```python
from build123d import *

# Parameters (mm, degrees)
F0_W     = 12.4
F0_H     = 29.8
F1_DEPTH = 12
F2_W     = 58.4
F2_H     = 12
F2_R     = 2.5
F3_DEPTH = 5
F4_R     = 5
F5_R     = 5
F6_R     = 5
F7_R     = 4.75
F8_DEPTH = 2
F9_R     = 1
F10_R    = 5


# Not quite as in the source:
# - a feature names something its author has since deleted; it is built from what else it names


with BuildPart() as f1:
    # F0 (on Top) → F1 (new body)
    with BuildSketch(Plane.XY):
        with BuildLine():
            ThreePointArc((-8.2, 0), (0, 8.2), (8.2, 0))
            Line((8.2, 0), (11.2, 0))
            Line((11.2, 0), (11.2, 52))
            Line((11.2, 52), (0, 52))
            Line((0, 52), (-11.2, 52))
            Line((-11.2, 52), (-11.2, 0))
            Line((-11.2, 0), (-8.2, 0))
        make_face()
        with Locations((0, 30.1)):
            Rectangle(F0_W, F0_H, mode=Mode.SUBTRACT)
        with BuildLine():
            Line((11.2, 0), (8.2, 0))
            ThreePointArc((8.2, 0), (0, -8.2), (-8.2, 0))
            Line((-8.2, 0), (-11.2, 0))
            Line((-11.2, 0), (-11.2, -12.2))
            Line((-11.2, -12.2), (0, -12.2))
            Line((0, -12.2), (11.2, -12.2))
            Line((11.2, -12.2), (11.2, 0))
        make_face()
        with BuildLine():
            Line((11.2, 0), (8.2, 0))
            ThreePointArc((8.2, 0), (0, -8.2), (-8.2, 0))
            Line((-8.2, 0), (-11.2, 0))
            Line((-11.2, 0), (-11.2, -12.2))
            Line((-11.2, -12.2), (0, -12.2))
            Line((0, -12.2), (11.2, -12.2))
            Line((11.2, -12.2), (11.2, 0))
        make_face()
    extrude(amount=F1_DEPTH)

    # F2 (on face) → F3 (join)
    with BuildSketch(Plane(origin=(0, 52, 0), x_dir=(-1, 0, 0), z_dir=(0, 1, 0))):
        with Locations((0, 6)):
            Rectangle(F2_W, F2_H)
        with Locations((-21.7, 6)):
            Circle(F2_R, mode=Mode.SUBTRACT)
        with Locations((21.7, 6)):
            Circle(F2_R, mode=Mode.SUBTRACT)
    extrude(amount=F3_DEPTH)

    # F4
    f4_edges = [f1.edges().sort_by_distance(p)[0] for p in [
        (-11.2, -12.2, 6),
        (11.2, -12.2, 6),
    ]]
    fillet(f4_edges, radius=F4_R)

    # F5
    f5_edges = [f1.edges().sort_by_distance(p)[0] for p in [
        (11.2, 52, 6),
        (-11.2, 52, 6),
    ]]
    fillet(f5_edges, radius=F5_R)

    # F6
    f6_edges = [f1.edges().sort_by_distance(p)[0] for p in [
        (-29.2, 54.5, 12),
        (-29.2, 54.5, 0),
        (29.2, 54.5, 0),
        (29.2, 54.5, 12),
    ]]
    fillet(f6_edges, radius=F6_R)

    # F7 (on face) → F8 (cut)
    with BuildSketch(Plane.XZ.offset(-52)):
        with Locations((21.7, 6)):
            Circle(F7_R)
        with Locations((-21.7, 6)):
            Circle(F7_R)
    extrude(amount=-F8_DEPTH, mode=Mode.SUBTRACT)

    # F9
    f9_edges = [f1.edges().sort_by_distance(p)[0] for p in [
        (8.2, 0, 12),
    ]]
    fillet(f9_edges, radius=F9_R)

    # F10
    f10_edges = [f1.edges().sort_by_distance(p)[0] for p in [
        (-6.2, 45, 6),
        (6.2, 45, 6),
        (-6.2, 15.2, 6),
        (6.2, 15.2, 6),
    ]]
    fillet(f10_edges, radius=F10_R)


solid = f1.part
```
Can you work these out from the model? Positions are in its coordinate system, mm. A direction names the side the tool comes from. Coordinates: 2 decimals unless noted, no trailing zeros. Loops run counter-clockwise (first coordinate to the right, second up) from the corner with the lowest first, then second, coordinate; pieces in that order, holes last. Notation, with made-up numbers: (57.5, 79.25) - (75.5, 79.25) arc R33 ccw to (75.5, 112.25) - close; hole circle Ø1 at (23.25, 73.25). An arc over 180 degrees is marked (long way). Answer as CSV lines item,"result". Start each with the question number.
1) I need wall thicknesses on line 1 (X direction, y = 55.2, z = 6); line 2 (Y direction, x = 0, z = 2.75); line 3 (X direction, y = 31, z = 8.5). Which ranges of each line are inside material? Lowest first, please. Write a range as from..to.
2) Suppose I cut it at B-B (x = -21.7). Please give me the cut outline in (y, z).
3) Suppose I cut it at D-D (z = 6). Count the separate pieces of the cut face and the enclosed holes in it, plus the area to 3 significant figures.
4) Thinking about a two-plate mould opening in Z: for faces 5 (the cylindrical face through (27.7, 54.54, 1.43)), 6 (the flat face through (-6.2, 30, 6)), 7 (the flat face through (-19.7, 54, 4)), which applies, pulls with the +Z half, pulls with the -Z half, needs draft (parallel to the pull), parting line crosses it, or undercut?
5) For pin 1 (6 mm diameter, centred on y = 13, z = 7, fed in from +X); pin 2 (6.5 mm diameter, centred on x = -21.7, z = 6, fed in from -Y); pin 3 (3 mm diameter, centred on x = -6, y = 20.5, fed in from -Z); pin 4 (5 mm diameter, centred on x = 10, z = 2.5, fed in from -Y), each with a flat end and sliding along its axis, tell me the tip position at first contact or that it passes through.
6) Which directions (+Z, -Z, +X, -X, +Y, -Y) give clear straight access to the entire face, cutting with the end or side of a thin tool? Please do faces 1 (the flat face through (24, 54, 4)), 2 (the cylindrical face through (4.7, 43.57, 6.08)), 3 (the flat face through (11.2, 20, 6)), 4 (the flat face through (-11.2, 20, 6)).
7) Suppose I cut it at A-A (x = 0). Please give me the cut outline in (y, z).
8) Suppose I cut it at C-C (y = 29.5). Please give me the cut outline in (x, z).
Check result:
1,line 1,"x = -29.2..-24.2, -19.2..19.2, 24.2..29.2"
1,line 2,"y = -12.2..-8.2, 8.2..15.2, 45..57"
1,line 3,"x = -11.2..-6.2, 6.2..11.2"
2,outline,"(52, 0) - (57, 0) - (57, 3.5) - (54, 3.5) - (54, 1.25) - (52, 1.25) - close; (52, 10.75) - (54, 10.75) - (54, 8.5) - (57, 8.5) - (57, 12) - (52, 12) - close"
3,separate pieces,"3"
3,enclosed holes,"2"
3,area,"1,100 mm²"
4,face 5,"pulls with the -Z half"
4,face 6,"needs draft"
4,face 7,"undercut"
5,pin 1,"stops at x = 11.2"
5,pin 2,"stops at y = 54"
5,pin 3,"stops at z = 0"
5,pin 4,"stops at y = -12.03"
6,face 1,"-Y"
6,face 2,"+Z, -Z"
6,face 3,"+Z, -Z, +X, -Y"
6,face 4,"+Z, -Z, -X, -Y"
7,outline,"(-12.2, 0) - (-8.2, 0) - (-8.2, 11) arc R1 ccw to (-9.2, 12) - (-12.2, 12) - close; (8.2, 0) - (15.2, 0) - (15.2, 12) - (9.2, 12) arc R1 ccw to (8.2, 11) - close; (45, 0) - (57, 0) - (57, 12) - (45, 12) - close"
8,outline,"(-11.2, 0) - (-6.2, 0) - (-6.2, 12) - (-11.2, 12) - close; (6.2, 0) - (11.2, 0) - (11.2, 12) - (6.2, 12) - close"
